Check sheet for the drawn part. Datum: minimum x, y, z corner. Units: mm. A direction names the side the tool comes from. Give positions to 0.01 mm unless a question says otherwise; leave off trailing zeros. Write each loop counter-clockwise with the first axis right and the second up, starting at its lowest first coordinate (ties: lowest second). Pieces come first, ordered by that corner, then holes.
(1) Tool access check on the marked faces 1, 2 and 3. Record the directions out of +Z, -Z, +X, -X, +Y, -Y that give a thin tool (end or side, any length) a straight path to the whole face; none if there is none.
(2) Cross-section at B-B (y = 36). Record the boundary of the cut face in (x, z), and give its area (3 significant figures).
(3) Cross-section at A-A (x = 27). Record the boundary of the cut face in (y, z).
(4) Cross-section at C-C (z = 16). Record the boundary of the cut face in (x, y).
(5) Cross-section at D-D (y = 17). Record the boundary of the cut face in (x, z).
(6) Depth check by flat-ended pin: P1, Ø5, axis at x = 24.5, y = 10.5, coming from the +Z side; P2, Ø9.5, axis at y = 37.5, z = 21, coming from the +X side; P3, Ø9.5, axis at x = 20.5, z = 24.5, coming from the +Y side. Enter the tip coordinate at first touch or a pass-through.
(7) Thickness scan on line 1 along Z through (x, y) = (27, 3); line 2 along Y through (x, z) = (15.5, 24.5). Record the ranges inside material, lowest first.
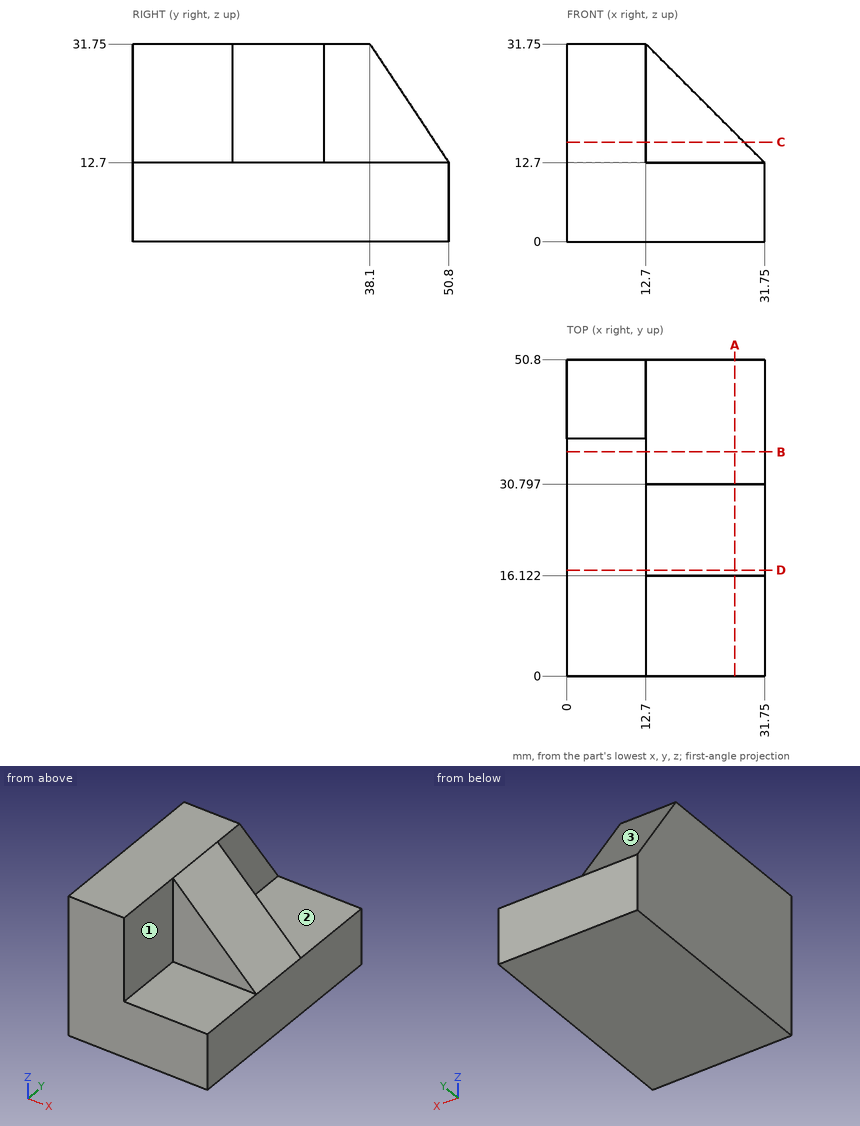
Reply:
1. face 1: +Z, +X, -Y
1. face 2: +Z, +X, +Y
1. face 3: +Z, +X, -X, +Y
2. outline: (0, 0) - (31.75, 0) - (31.75, 12.7) - (12.7, 12.7) - (12.7, 31.75) - (0, 31.75) - close
2. area: 645 mm2
3. outline: (0, 0) - (50.8, 0) - (50.8, 12.7) - (30.8, 12.7) - (30.8, 17.45) - (16.12, 17.45) - (16.12, 12.7) - (0, 12.7) - close
4. outline: (0, 0) - (12.7, 0) - (12.7, 16.12) - (28.45, 16.12) - (28.45, 30.8) - (12.7, 30.8) - (12.7, 48.6) - (0, 48.6) - close
5. outline: (0, 0) - (31.75, 0) - (31.75, 12.7) - (12.7, 31.75) - (0, 31.75) - close
6. P1: stops at z = 12.7
6. P2: stops at x = 12.7
6. P3: stops at y = 30.8
7. line 1: z = 0 to 12.7
7. line 2: y = 16.12 to 30.8
